The model under review builds one solid part; all positions refer to its coordinate system, in mm. A direction names the side the tool comes from. Round coordinates to 2 decimals unless told otherwise and drop trailing zeros. Write each loop counter-clockwise with the first axis right and the second up, starting at its lowest first coordinate (ties: lowest second). Pieces come first, ordered by that corner, then holes.
Item 1: Draft analysis for pull direction X (two halves, no side actions). For faces 3 (the face through (-0.9, 8.95, -2.86)), 4 (the face through (0, -0.289, 0)), 5 (the face through (0, 8.961, 0)), state which applies: +X half, -X half, draft (parallel to the pull), parting line (faces both ways), or undercut.
Item 2: Machinability: for faces 1 (the face through (2, 9.711, 0)), 2 (the face through (-0.45, 4.05, -1.43)), which of the approach directions +Z, -Z, +X, -X, +Y, -Y give a long, thin tool a straight path to every point of the face, cutting with its end or side? Answer none if there is none.
Item 3: Add section A-A (z = 0). Give the boundary of the cut face in (x, y).
Item 4: Add section C-C (y = 7). Give the boundary of the cut face in (x, z), plus the area to 3 significant figures.
Item 5: Add section D-D (z = 1.8). Give the boundary of the cut face in (x, y).
Item 6: To check wall thickness, follow L1, parallel to Y at x = 0.8, z = 2.1; L2, parallel to X at y = 5, z = 1.1; L3, parallel to Y at x = 0.1, z = 1.1. State the ranges of each line that lie inside material, in increasing order.
Item 7: Clearance check with flat-ended pins moving along their axes: pin 1 Ø3 at (x, z) = (1, 1) entering from -Y; pin 2 Ø3 at (y, z) = (6, -1.5) entering from -X; pin 3 Ø1 at (x, z) = (-1.5, -1) entering from -Y; pin 4 Ø1.5 at (y, z) = (2.5, 2) entering from -X. State where each tip first meets the part, or that it passes through.
Item 8: Add section B-B (x = 0). Give the boundary of the cut face in (y, z).
```python
from build123d import *

# Parameters (mm, degrees)
ENL_V_MAT_EXTRU_1_DEPTH      = 11.597633257
ENL_V_MAT_EXTRU_1_DEPTH_BACK = 11.597633257
ESQUISSE2_W                  = 1.5
ESQUISSE2_H                  = 0.75


with BuildPart() as part:
    # Esquisse1 → Révolution1 (revolve)
    with BuildSketch(Plane.XY, mode=Mode.PRIVATE) as r_volution1_sk:
        Polygon((0, 0), (0, 9.711324865), (3, 9.711324865), (3, 8.211324865), (1.5, 8.211324865), (1.5, 0), (1, -0.288675135), (0, -0.288675135), align=None)
    revolve(r_volution1_sk.sketch.rotate(Axis((0, 0, 0), (0, 1, 0)), 90), axis=Axis((0, 0, 0), (0, 1, 0)))

    # Esquisse2 → Enlèv. mat.-Extru.1 (cut, two sides: drawn at the far end of the back side and taken through both)
    with BuildSketch(Plane.XY.offset(-ENL_V_MAT_EXTRU_1_DEPTH_BACK)):
        with Locations((0, 9.336324865)):
            Rectangle(ESQUISSE2_W, ESQUISSE2_H)
    extrude(amount=ENL_V_MAT_EXTRU_1_DEPTH + ENL_V_MAT_EXTRU_1_DEPTH_BACK, mode=Mode.SUBTRACT)


solid = part.part
```
Numbers:
1. face 3: parting line
1. face 4: draft
1. face 5: undercut
2. face 1: +Z, -Z, +X, -X, +Y
2. face 2: -Y
3. outline: (-3, 8.21) - (-1.5, 8.21) - (-1.5, 0) - (-1, -0.29) - (1, -0.29) - (1.5, 0) - (1.5, 8.21) - (3, 8.21) - (3, 9.71) - (0.75, 9.71) - (0.75, 8.96) - (-0.75, 8.96) - (-0.75, 9.71) - (-3, 9.71) - close
4. outline: circle Ø3 at (0, 0)
4. area: 7.07 mm2
5. outline: (-2.4, 8.21) - (2.4, 8.21) - (2.4, 9.71) - (0.75, 9.71) - (0.75, 8.96) - (-0.75, 8.96) - (-0.75, 9.71) - (-2.4, 9.71) - close
6. L1: y = 8.21 to 9.71
6. L2: x = -1.02 to 1.02
6. L3: y = -0.23 to 8.96
7. pin 1: stops at y = -0.29
7. pin 2: stops at x = -1.5
7. pin 3: stops at y = -0.11
7. pin 4: stops at x = -0.83
8. outline: (-0.29, -1) - (0, -1.5) - (8.21, -1.5) - (8.21, -3) - (8.96, -3) - (8.96, 3) - (8.21, 3) - (8.21, 1.5) - (0, 1.5) - (-0.29, 1) - close
